Autodesk Inventor part; units mm, degrees
ref_plane "Work Plane1" through (0, 0, -15) normal (0, 0, 1) x (1, 0, 0)
ref_plane "YZ Plane" through (0, 0, 0) normal (1, 0, 0) x (0, 1, 0)
ref_plane "XZ Plane" through (0, 0, 0) normal (0, 1, 0) x (-1, 0, 0)
sketch "Sketch1" plane through (0, 0, 0) normal (0, 0, 1) x (1, 0, 0)
  line L0 (0, 0) -> (25, 0)
  line L1 (25, 0) -> (25, 40)
  line L2 (25, 40) -> (0, 40)
  line L3 (0, 40) -> (0, 0)
  dimension "d1" = 25
  dimension "d2" = 40
  dimension "d3" = 25
extrude "Extrusion1" add sketch "Sketch1" against normal blind 30
sketch "Sketch2" plane through (25, 0, 0) normal (1, 0, 0) x (0, 0, -1)
  line L0 (0, 0) -> (30, 0)
  circle A0 centre (15, 6.56) radius 2.46
extrude "Extrusion2" cut sketch "Sketch2" against normal blind 30
sketch "Sketch3" plane through (0, 0, 0) normal (-1, 0, 0) x (0, 0, 1)
  line L0 (0, 0) -> (-30, 0)
  line L1 (-25.05, 0) -> (-4.95, 0)
  line L2 (-4.95, 0) -> (-4.95, 33.12)
  line L3 (-4.95, 33.12) -> (-25.05, 33.12)
  line L4 (-25.05, 33.12) -> (-25.05, 0)
  dimension "d11" = 20.1
extrude "Extrusion3" cut sketch "Sketch3" against normal blind 20
sketch "Sketch4" plane through (0, 0, 0) normal (0, -1, 0) x (1, 0, 0)
  line L0 (20, -4.95) -> (20, -25.05)
  line L1 (20, -15) -> (25, -15)
  line L2 (25, 0) -> (25, -30)
  line L3 (20, -8.025) -> (25, -8.025)
  line L4 (25, -8.025) -> (25, -21.975)
  line L5 (25, -21.975) -> (20, -21.975)
  line L6 (20, -21.975) -> (20, -8.025)
  line L7 (20, -8.025) -> (25, -21.975) construction
  line L8 (25, -8.025) -> (20, -21.975) construction
  line L9 (25, -12.54) -> (25, -17.46)
  point P0 (0, 0)
  point P1 (22.5, -15)
  dimension "d14" = 13.95
extrude "Extrusion4" add sketch "Sketch4" along normal blind 15
sketch "Sketch5" plane through (20, 0, 0) normal (-1, 0, 0) x (0, 0, 1)
  circle A0 centre (-15, 6.56) radius 2.46
  circle A1 centre (-15, 6.56) radius 4.7025
  circle A2 centre (-15, 6.56) radius 2.46
  circle A3 centre (-15, 6.56) radius 2.46
  point P0 (0, 0)
  dimension "d17" = 9.405
extrude "Extrusion5" cut sketch "Sketch5" against normal blind 2.1
sketch "Sketch6" plane through (25, 0, 0) normal (1, 0, 0) x (0, 0, -1)
  circle A0 centre (15, 6.56) radius 4.7025
  line L0 (15, 6.56) -> (15, 23.56)
  circle A1 centre (15, 23.56) radius 2.46
  point P0 (0, 0)
  dimension "d20" = 17
  dimension "d21" = 4.92
extrude "Extrusion6" cut sketch "Sketch6" against normal blind 10 contours A1
sketch "Sketch7" plane through (20, 0, 0) normal (-1, 0, 0) x (0, 0, 1)
  circle A0 centre (-15, 23.56) radius 2.46
  circle A1 centre (-15, 23.56) radius 4.7025
  point P0 (0, 0)
  dimension "d24" = 9.405
extrude "Extrusion7" cut sketch "Sketch7" against normal blind 2.1
sketch "Sketch9" plane through (25, 0, 0) normal (1, 0, 0) x (0, 0, -1)
  circle A0 centre (15, 6.56) radius 2.46
  circle A1 centre (15, 6.56) radius 2.46
  circle A2 centre (15, 23.56) radius 2.46
  circle A3 centre (15, 23.56) radius 2.46
  line L0 (30, 40) -> (30, 0)
  line L1 (30, 0) -> (30, 40)
  line L2 (30, 40) -> (0, 40)
  line L3 (0, 40) -> (0, 0)
  line L4 (0, 0) -> (8.025, 0)
  line L5 (21.975, 0) -> (21.975, -15)
  line L6 (21.975, -15) -> (8.025, -15)
  line L7 (8.025, -15) -> (8.025, 0)
  line L8 (0, 0) -> (8.025, 0)
  line L9 (21.975, 0) -> (30, 0)
extrude "Extrusion8" add sketch "Sketch9" along normal blind 5
sketch "Sketch10" plane through (0, 40, 0) normal (0, 1, 0) x (1, 0, 0)
  line L0 (0, 30) -> (30, 30)
  line L1 (30, 0) -> (0, 0)
  line L2 (0, 30) -> (30, 30)
  line L3 (30, 30) -> (30, 0)
  line L4 (30, 0) -> (0, 0)
  line L5 (0, 0) -> (0, 30)
extrude "Extrusion9" add sketch "Sketch10" along normal blind 30
sketch "Sketch12" plane through (30, 0, 0) normal (1, 0, 0) x (0, 0, -1)
  circle A0 centre (15, 6.56) radius 2.46
  line L0 (15, 6.56) -> (15, 15.06)
  circle A1 centre (15, 15.06) radius 2.525
  point P0 (0, 0)
  dimension "d31" = 8.5
  dimension "d33" = 5.05
extrude "Extrusion10" cut sketch "Sketch12" against normal blind 30 contours A1
sketch "Sketch14" plane through (0, 0, 0) normal (0, 0, 1) x (1, 0, 0)
  line L0 (30, 70) -> (0, 70)
  line L1 (0, 70) -> (0, 85)
  line L2 (-15, 100) -> (-23, 100)
  line L3 (30, 0) -> (30, 70)
  line L4 (30, 118) -> (30, 70)
  arc A0 (0, 85) -> (-15, 100) centre (-15, 85) ccw
  line L5 (30, 105) -> (30, 100)
  line L6 (-18, 134) -> (-23, 136)
  line L7 (-18, 102) -> (-23, 100)
  line L8 (-18, 102) -> (-13, 118)
  line L9 (-13, 118) -> (-18, 134)
  line L10 (15, 136) -> (30, 118)
  line L11 (-23, 136) -> (15, 136)
  point P0 (0, 0)
  point P1 (0, 100)
  dimension "d47" = 30
  dimension "d54" = 15
extrude "Extrusion12" add sketch "Sketch14" against normal blind 30
sketch "Sketch15" plane through (0, 0, -25.05) normal (-1, 0, 0) x (0, 0, 1)
  line L0 (0, 33.12) -> (20.1, 33.12)
  line L1 (20.1, 33.12) -> (20.1, 0)
  line L2 (0, 33.12) -> (20.1, 33.12)
  line L3 (20.1, 33.12) -> (20.1, 31.1)
  line L4 (20.1, 31.1) -> (0, 31.1)
  line L5 (0, 31.1) -> (0, 33.12)
  point P0 (25.05, 0)
  dimension "d57" = 2.02
extrude "Extrusion13" add sketch "Sketch15" against normal blind 20
sketch "Sketch22" plane through (0, 0, 0) normal (0, 0, 1) x (1, 0, 0)
  line L0 (-15, 100) -> (-23, 100)
  line L1 (-15, 100) -> (-23, 100)
  line L2 (-23, 100) -> (-18, 102)
  line L3 (-23, 100) -> (-18, 102)
  line L4 (-18, 102) -> (-13, 118)
  line L5 (-18, 102) -> (-13, 118)
  line L6 (-13, 118) -> (-18, 134)
  line L7 (-13, 118) -> (-18, 134)
  line L8 (-18, 134) -> (-23, 136)
  line L9 (-18, 134) -> (-23, 136)
  line L10 (-23, 136) -> (15, 136)
  line L11 (-23, 136) -> (15, 136)
  line L12 (15, 136) -> (30, 118)
  line L13 (15, 136) -> (30, 118)
  line L14 (30, 118) -> (30, 78)
  line L15 (30, 0) -> (30, 118)
  line L16 (30, 78) -> (0, 78)
  arc A0 (0, 85) -> (-15, 100) centre (-15, 85) ccw
  line L17 (0, 78) -> (0, 85)
  arc A1 (0, 85) -> (-15, 100) centre (-15, 85) ccw
  point P0 (0, 0)
  dimension "d82" = 40
extrude "Extrusion14" add sketch "Sketch22" along normal blind 30
ref_plane "Work Plane1" through (0, 0, -15) normal (0, 0, 1) x (1, 0, 0)
mirror "Mirror1" about plane through (0, 0, -15) normal (0, 0, 1) of "Extrusion14"
properties part number "rec_a_32mm_x_90mm"
Verification items for the finished model (mm, model axes). A direction names the side the tool comes from. Give positions to 0.01 mm unless a question says otherwise; leave off trailing zeros. Write each loop counter-clockwise with the first axis right and the second up, starting at its lowest first coordinate (ties: lowest second). Pieces come first, ordered by that corner, then holes.
(1) Mould release check, pull along Z, two halves, no side actions. Record for faces 6 (the face through (25.995, 24.502, -17.272)), 7 (the face through (9, 107, 30)), 8 (the face through (25, -7, -21.975)): +Z half, -Z half, draft (parallel to the pull), parting line (faces both ways), or undercut.
(2) Cross-section at B-B (y = 6.56). Enter the section's corners in (x, z), plus the area to 3 significant figures.
(3) Cross-section at D-D (x = 3). Enter the section's corners in (y, z).
(4) Cross-section at C-C (z = -43). Enter the section's corners in (x, y).
(5) Cross-section at A-A (x = -16.5). Enter the section's corners in (y, z).
(6) Gauge pin test, flat ends, axial feed: pin 1 (9 mm diameter, centred on x = 18, y = 30, fed in from -Z); pin 2 (8 mm diameter, centred on y = 6.56, z = -15, fed in from -X); pin 3 (7.5 mm diameter, centred on y = 25.5, z = -14.5, fed in from -X); pin 4 (4 mm diameter, centred on y = 23.56, z = -15, fed in from +X). Record the tip position at first contact, or that the pin passes through.
(7) Access from +Z, -Z, +X, -X, +Y, -Y to the whole of each face (thin tool, end or side, straight path). Record for faces 1 (the face through (22.1, 21.5, -13)), 2 (the face through (-20.5, 101, -14.4)), 3 (the face through (15, 40, 0)), 4 (the face through (15, 40, -30)), 5 (the face through (10, 31.1, -15)).
(8) Material ranges on line 1 (Y direction, x = 27.75, z = -15) (3 decimals); line 2 (Z direction, x = 26.75, y = 23.56); line 3 (Y direction, x = 27, z = -15) (3 decimals), recorded low to high.
Worked out:
1. face 6: undercut
1. face 7: +Z half
1. face 8: -Z half
2. outline: (0, -30) - (30, -30) - (30, -17.46) - (22.1, -17.46) - (22.1, -19.7) - (20, -19.7) - (20, -25.05) - (0, -25.05) - close; (0, -4.95) - (20, -4.95) - (20, -10.3) - (22.1, -10.3) - (22.1, -12.54) - (30, -12.54) - (30, 0) - (0, 0) - close
2. area: 439 mm2
3. outline: (0, -30) - (78, -30) - (78, -60) - (136, -60) - (136, 30) - (78, 30) - (78, 0) - (0, 0) - (0, -4.95) - (31.1, -4.95) - (31.1, -25.05) - (0, -25.05) - close
4. outline: (-23, 100) - (-15, 100) arc R15 cw to (0, 85) - (0, 78) - (30, 78) - (30, 118) - (15, 136) - (-23, 136) - (-18, 134) - (-13, 118) - (-18, 102) - close
5. outline: (100, -60) - (106.8, -60) - (106.8, 30) - (100, 30) - close; (129.2, -60) - (136, -60) - (136, 30) - (129.2, 30) - close
6. pin 1: stops at z = -30
6. pin 2: stops at x = 22.1
6. pin 3: stops at x = 20
6. pin 4: passes through
7. face 1: -X
7. face 2: +Z, -Z, -X
7. face 3: +Z, +X, -X, -Y
7. face 4: -Z, +X, -X, -Y
7. face 5: -X, -Y
8. line 1: y = -15 to 4.1, 9.02 to 12.535, 17.585 to 21.1, 26.02 to 120.7
8. line 2: z = -30 to -17.46, -12.54 to 0
8. line 3: y = -15 to 4.1, 9.02 to 12.535, 17.585 to 21.1, 26.02 to 121.6
